The listing builds one solid part. Answer for the finished solid, in the listing's coordinates (mm). A direction names the side the tool comes from. Coordinates: 2 decimals unless noted, no trailing zeros. Order: outer loops, then holes, each group sorted by start corner. A loop starts at its lowest first (then second) coordinate and runs counter-clockwise, first axis right, second up. Notation, with made-up numbers: (35.25, 41.5) -> (51.25, 41.5) arc R24 ccw to (51.25, 56.5) -> close; hole circle Ø1 at (-19, 67). An arc over 180 degrees is marked (long way). Write each question's results on one line, items separated by ' | '. Start each with the question number.
(1) The part is cut by section D-D, the plane y = 158.5. Give the vertices of the cut face in (x, z), then the cut area to 3 significant figures.
(2) Given pin 1 (1.5 mm diameter, centred on y = 131, z = 349, fed in from +X); pin 2 (8 mm diameter, centred on x = 384, z = 188.5, fed in from -Y); pin 3 (8 mm diameter, centred on x = 75.5, y = 191.5, fed in from +Z), each flat-ended and moving along its own axis, determine where each tip first touches the part or whether it passes through.
(3) A tool of negligible diameter and unlimited length cuts with its end or side. For faces 1 (the face through (-533.126, 66, -29)), 2 (the face through (125.834, 215.1, 537.734)), from which of +Z, -Z, +X, -X, +Y, -Y can it reach the whole face along a straight path? Write none if from no direction.
(4) Straight lines are drawn through the part: L1, parallel to Z at x = 539.5, y = 36; L2, parallel to X at y = 70.5, z = 238.5; L3, parallel to Y at x = 338.5, z = -47.5. For each, find the intervals that lie inside material, in ascending order.
(5) The part is cut by section A-A, the plane y = 77. Give the vertices of the cut face in (x, z), then the cut area to 3 significant figures.
(6) The part is cut by section C-C, the plane x = 538. Give the vertices of the cut face in (y, z), then the cut area to 3 significant figures.
(7) The part is cut by section B-B, the plane z = -169. Give the vertices of the cut face in (x, y), then the cut area to 3 significant figures.
(8) Determine the mould class of faces 3 (the face through (766.874, 66, -29)), 4 (the face through (108, 66, 577.657)), 5 (the face through (108, 66, 587.657)) for opening direction Z: +Z half, -Z half, draft (parallel to the pull), parting line (faces both ways), or undercut.
```python
from build123d import *

# Parameters (mm, degrees)
SKETCH2_W           = 1300
SKETCH2_H           = 1250
BOSS_EXTRUDE1_DEPTH = 250
FILLET2_R           = 150
SHELL3_T            = -10


with BuildPart() as part:
    # Sketch2 → Boss-Extrude1 (new body)
    with BuildSketch(Plane(origin=(0, 17.2, 0), x_dir=(1, 0, 0), z_dir=(0, 1, 0))):
        with Locations((116.873880354, 37.343378517)):
            Rectangle(SKETCH2_W, SKETCH2_H)
    extrude(amount=BOSS_EXTRUDE1_DEPTH)

    # Fillet2
    fillet2_edges = [part.edges().sort_by_distance(p)[0] for p in [
        (116.873880354, 267.2, 587.656621483),
        (766.873880354, 267.2, -37.343378517),
        (116.873880354, 267.2, -662.343378517),
        (-533.126119646, 267.2, -37.343378517),
    ]]
    fillet(fillet2_edges, radius=FILLET2_R)

    # Shell3
    shell3_openings = [part.faces().sort_by_distance(p)[0] for p in [
        (116.873880354, 17.2, -37.343378517),
    ]]
    offset(amount=SHELL3_T, openings=shell3_openings)


solid = part.part
```
Established:
1) outline: (-527.33, -656.55) -> (761.08, -656.55) -> (761.08, 581.86) -> (-527.33, 581.86) -> close; hole (-516.9, -646.11) -> (750.64, -646.11) -> (750.64, 571.43) -> (-516.9, 571.43) -> close | area: 52,300 mm^2
2) pin 1: stops at x = 766.31 | pin 2: stops at y = 257.2 | pin 3: stops at z = 570.16
3) face 1: +Z, -Z, -X, +Y, -Y | face 2: -Y
4) L1: z = -662.34 to -652.34, 577.66 to 587.66 | L2: x = -533.13 to -523.13, 756.87 to 766.87 | L3: y = 257.2 to 267.2
5) outline: (-533.13, -662.34) -> (766.87, -662.34) -> (766.87, 587.66) -> (-533.13, 587.66) -> close; hole (-523.13, -652.34) -> (756.87, -652.34) -> (756.87, 577.66) -> (-523.13, 577.66) -> close | area: 50,600 mm^2
6) outline: (17.2, -662.34) -> (117.2, -662.34) arc R150 ccw to (267.2, -512.34) -> (267.2, 437.66) arc R150 ccw to (117.2, 587.66) -> (17.2, 587.66) -> (17.2, 577.66) -> (117.2, 577.66) arc R140 cw to (257.2, 437.66) -> (257.2, -512.34) arc R140 cw to (117.2, -652.34) -> (17.2, -652.34) -> close | area: 16,100 mm^2
7) outline: (-533.13, 17.2) -> (-523.13, 17.2) -> (-523.13, 117.2) arc R140 cw to (-383.13, 257.2) -> (616.87, 257.2) arc R140 cw to (756.87, 117.2) -> (756.87, 17.2) -> (766.87, 17.2) -> (766.87, 117.2) arc R150 ccw to (616.87, 267.2) -> (-383.13, 267.2) arc R150 ccw to (-533.13, 117.2) -> close | area: 16,600 mm^2
8) face 3: draft | face 4: undercut | face 5: +Z half
